```python
from build123d import *

# Parameters (mm, degrees)
SKETCH6_R          = 22.921214
SKETCH6_R_2        = 20.381214
CUT_EXTRUDE2_DEPTH = 1.3462


with BuildPart() as part:
    # Sketch1 → Revolve1 (revolve)
    with BuildSketch(Plane.XY):
        Polygon((0, 35.56), (6.35, 35.56), (6.35, 24.13), (70.9600054, 24.13), (70.9600054, 5.999988), (60.8000054, 5.999988), (60.8000054, 12.7), (48.1000054, 12.7), (48.1000054, 15.24), (22.7000054, 15.24), (22.7000054, 16.002), (12.7, 16.002), (12.7, 18.542), (0, 18.542), align=None)
    revolve(axis=Axis((0, 0, 0), (1, 0, 0)))

    # Sketch6 → Cut-Extrude2 (cut)
    with BuildSketch(Plane.ZY):
        Circle(SKETCH6_R)
        Circle(SKETCH6_R_2, mode=Mode.SUBTRACT)
    extrude(amount=-CUT_EXTRUDE2_DEPTH, mode=Mode.SUBTRACT)


solid = part.part
```
Input: part model. Units: mm. Frame: model coordinates. A direction names the side the tool comes from. Round coordinates to 2 decimals unless told otherwise and drop trailing zeros. Loops run counter-clockwise (first coordinate to the right, second up) from the corner with the lowest first, then second, coordinate; pieces in that order, holes last.
1) Material intervals for line 1 (Z direction, x = 8.5, y = 0); line 2 (Z direction, x = 51, y = 0); line 3 (X direction, y = 19, z = -26), sorted ascending.
Ans:
line 1: z = -24.13 to -18.54, 18.54 to 24.13
line 2: z = -24.13 to -12.7, 12.7 to 24.13
line 3: x = 0 to 6.35
2) Set-up query: faces 4 (the flat face through (0, 0.5, -23.2)), 5 (the cylindrical face through (17.63, -3.47, -15.62)). Return all of +Z, -Z, +X, -X, +Y, -Y with unobstructed straight access to the full face (end or side cutting, diameter ignored); none if empty.
Ans:
face 4: +Z, -Z, -X, +Y, -Y
face 5: -X
3) Section query A-A on x = 11.5. Return the cut outline in (y, z).
Ans:
outline: circle Ø48.26 at (0, 0); hole circle Ø37.08 at (0, 0)
4) Section query D-D on x = 28.5. Return the cut outline in (y, z), plus the area to 3 significant figures.
Ans:
outline: circle Ø48.26 at (0, 0); hole circle Ø30.48 at (0, 0)
area: 1,100 mm2
5) Section query B-B on y = 14. Return the cut outline in (x, z), plus the area to 3 significant figures.
Ans:
outline: (0, -32.69) - (6.35, -32.69) - (6.35, -19.65) - (70.96, -19.65) - (70.96, 19.65) - (6.35, 19.65) - (6.35, 32.69) - (0, 32.69) - (0, 18.15) - (1.35, 18.15) - (1.35, 14.81) - (0, 14.81) - (0, 12.16) - (12.7, 12.16) - (12.7, 7.75) - (22.7, 7.75) - (22.7, 6.02) - (48.1, 6.02) - (48.1, -6.02) - (22.7, -6.02) - (22.7, -7.75) - (12.7, -7.75) - (12.7, -12.16) - (0, -12.16) - (0, -14.81) - (1.35, -14.81) - (1.35, -18.15) - (0, -18.15) - close
area: 2,180 mm2
6) Pin query (flat end, axial travel): pin 1 (3 mm diameter, centred on x = 27, z = 4, fed in from +Y); pin 2 (8 mm diameter, centred on x = 25.5, y = -5, fed in from +Z); pin 3 (3 mm diameter, centred on x = 27.5, y = -19, fed in from -Z). Return the tip coordinate at first contact, or that it passes through.
Ans:
pin 1: stops at y = 24
pin 2: stops at z = 24.11
pin 3: stops at z = -16.61
7) Pull-direction query (Y, two-part tool) for faces 1 (the flat face through (6.35, 7.4, -23.2)), 2 (the cylindrical face through (39.107, 23.016, 7.248)), 3 (the flat face through (12.7, 6, 15)); classes: released by +Y, released by -Y, zero draft, split by the parting line, or undercut.
Ans:
face 1: zero draft
face 2: split by the parting line
face 3: undercut
